Autodesk Inventor part; units mm, degrees
ref_plane "YZ Plane" through (0, 0, 0) normal (1, 0, 0) x (0, 1, 0)
ref_plane "XZ Plane" through (0, 0, 0) normal (0, 1, 0) x (-1, 0, 0)
ref_plane "XY Plane" through (0, 0, 0) normal (0, 0, 1) x (1, 0, 0)
sketch "Sketch1" plane through (0, 0, 0) normal (0, 1, 0) x (-1, 0, 0)
  circle A0 centre (0, 0) radius 67.875
  circle A1 centre (0, 0) radius 64.25
  circle A2 centre (0, 0) radius 61.125
  circle A3 centre (0, 0) radius 9.5
  dimension "Absolute_Diameter" = 135.75
  dimension "Diameter_No_Outer_Lip" = 128.5
  dimension "Inner_Cylinder_Diameter" = 122.25
  dimension "Lip_Diameter" = 19
extrude "Extrusion1" add sketch "Sketch1" along normal blind 5 contours A0
extrude "Extrusion2" add sketch "Sketch1" along normal blind 75 contours A1
sketch "Sketch2" plane through (0, 75, 0) normal (0, 1, 0) x (1, 0, 0)
  circle A0 centre (0, 0) radius 64.25
  circle A1 centre (0, 0) radius 57.5
  dimension "Lip_Diameter_Out" = 128.5
  dimension "Inner_Lip_Diameter" = 115
extrude "Extrusion7" add sketch "Sketch2" against normal blind 5
chamfer "Chamfer1" distance 0.5 angle 45 2 edges at (64.25, 75, 0) (-57.5, 75, 0)
chamfer "Chamfer2" distance 0.5 angle 45 3 edges at (67.875, 5, 0) (67.875, 0, 0) (61.125, 0, 0)
sketch "Sketch3" plane through (0, 5, 0) normal (0, 1, 0) x (1, 0, 0)
  circle A0 centre (0, 0) radius 127.5
  circle A1 centre (-127.5, 0) radius 2
  circle A2 centre (-103.1497, -74.9426) radius 2
  circle A3 centre (-39.3997, -121.2597) radius 2
  circle A4 centre (39.3997, -121.2597) radius 2
  circle A5 centre (103.1497, -74.9426) radius 2
  circle A6 centre (127.5, 0) radius 2
  circle A7 centre (103.1497, 74.9426) radius 2
  circle A8 centre (39.3997, 121.2597) radius 2
  circle A9 centre (-39.3997, 121.2597) radius 2
  circle A10 centre (-103.1497, 74.9426) radius 2
  dimension "d27" = 255
  dimension "d28" = 4
  dimension "d31" = 360
extrude "Extrusion8" [suppressed]
sketch "Sketch4" plane through (0, 75, 0) normal (0, 1, 0) x (1, 0, 0)
  circle A0 centre (0, 0) radius 42.5
  circle A1 centre (0, 0) radius 37.5
  circle A2 centre (0, 0) radius 40
  circle A3 centre (-40, 0) radius 1
  circle A4 centre (-24.9396, -31.2733) radius 1
  circle A5 centre (8.9008, -38.9971) radius 1
  circle A6 centre (36.0388, -17.3553) radius 1
  circle A7 centre (36.0388, 17.3553) radius 1
  circle A8 centre (8.9008, 38.9971) radius 1
  circle A9 centre (-24.9396, 31.2733) radius 1
  dimension "d35" = 80
  dimension "d36" = 2
  dimension "d39" = 360
hole "Hole1" [suppressed]
properties part number "Cylinder  Segment - 08"
Source: CAD feature listing. Evaluate the final solid. Frame: model axes, mm. A direction names the side the tool comes from. Coordinates: 2 decimals unless noted, no trailing zeros. Loops run counter-clockwise (first coordinate to the right, second up) from the corner with the lowest first, then second, coordinate; pieces in that order, holes last. Notation, with made-up numbers: (-3, 36.25) -> (22, 36.25) arc R18 ccw to (22, 44.25) -> close; hole circle Ø7 at (63.25, -14). An arc over 180 degrees is marked (long way). Answer in a Markdown table with one row per item. Add a question column.
Q1. Contact query for flat-ended pins moving along their axis: pin 1 Ø5 at (y, z) = (11.5, 1.5) entering from -X; pin 2 Ø6 at (x, y) = (-26, 42) entering from -Z; pin 3 Ø12 at (x, y) = (-52.5, 45.5) entering from -Z. Output: stop coordinate, or through.
Q2. Section C-C on y = 52.5. Return the cut outline in (x, z) (3 decimals).
Q3. Ray query, line 1 along Z through (x, y) = (0, 71.4); line 2 along Z through (x, y) = (0, 50) (3 decimals); line 3 along X through (y, z) = (58.5, -20.5). Return the intervals inside material, ascending.
Q4. Section A-A on x = 0. Return the cut outline in (y, z) (3 decimals), and give its area (3 significant figures).
Q5. Section B-B on z = 0. Return the cut outline in (x, y) (3 decimals), and give its area (3 significant figures).
Q6. Pull-direction query (X, two-part tool) for faces 4 (the face through (13.93, 39.26, 62.72)), 5 (the face through (22, 70, 54)), 6 (the face through (-30, 0, -55)); classes: pulls with the +X half, pulls with the -X half, needs draft (parallel to the pull), parting line crosses it, or undercut.
Q7. Reachability of faces 1 (the face through (-60, 5, -25)), 2 (the face through (14.5, 75, -56.4)), 3 (the face through (13.25, 34.76, 59.67)) from +Z, -Z, +X, -X, +Y, -Y: full face, straight path, thin tool, end or side. Return the list, or none.
Computed values:
| question | item | result |
|---|---|---|
| 1 | pin 1 | stops at x = -64.25 |
| 1 | pin 2 | stops at z = -59.99 |
| 1 | pin 3 | stops at z = -44.34 |
| 2 | outline | circle Ø128.5 at (0, 0); hole circle Ø122.25 at (0, 0) |
| 3 | line 1 | z = -64.25 to -57.5, 57.5 to 64.25 |
| 3 | line 2 | z = -64.25 to -61.125, 61.125 to 64.25 |
| 3 | line 3 | x = -60.89 to -57.58, 57.58 to 60.89 |
| 4 | outline | (0, -67.375) -> (0.5, -67.875) -> (4.5, -67.875) -> (5, -67.375) -> (5, -64.25) -> (74.5, -64.25) -> (75, -63.75) -> (75, -58) -> (74.5, -57.5) -> (70, -57.5) -> (70, -61.125) -> (0.5, -61.125) -> (0, -61.625) -> close; (0, 61.625) -> (0.5, 61.125) -> (70, 61.125) -> (70, 57.5) -> (74.5, 57.5) -> (75, 58) -> (75, 63.75) -> (74.5, 64.25) -> (5, 64.25) -> (5, 67.375) -> (4.5, 67.875) -> (0.5, 67.875) -> (0, 67.375) -> close |
| 4 | area | 540 mm^2 |
| 5 | outline | (-67.875, 0.5) -> (-67.375, 0) -> (-61.625, 0) -> (-61.125, 0.5) -> (-61.125, 70) -> (-57.5, 70) -> (-57.5, 74.5) -> (-58, 75) -> (-63.75, 75) -> (-64.25, 74.5) -> (-64.25, 5) -> (-67.375, 5) -> (-67.875, 4.5) -> close; (57.5, 70) -> (61.125, 70) -> (61.125, 0.5) -> (61.625, 0) -> (67.375, 0) -> (67.875, 0.5) -> (67.875, 4.5) -> (67.375, 5) -> (64.25, 5) -> (64.25, 74.5) -> (63.75, 75) -> (58, 75) -> (57.5, 74.5) -> close |
| 5 | area | 540 mm^2 |
| 6 | face 4 | parting line crosses it |
| 6 | face 5 | undercut |
| 6 | face 6 | needs draft |
| 7 | face 1 | +Y |
| 7 | face 2 | +Z, -Z, +X, -X, +Y |
| 7 | face 3 | -Y |
